The model under review builds one solid part; all positions refer to its coordinate system, in mm. A direction names the side the tool comes from. Coordinates: 2 decimals unless noted, no trailing zeros. Loops run counter-clockwise (first coordinate to the right, second up) from the corner with the lowest first, then second, coordinate; pieces in that order, holes last. Notation, with made-up numbers: M 39.25,-4.75 L 51.25,-4.75 A8 ccw 51.25,1.25 Z; hole C 14.25,-38.5 d3. An arc over 180 degrees is marked long. Use CSV: the item, a comma, the result in double quotes. Start each with the question number.
1. Tool access review of faces 4 (the cylindrical face through (-5.961, -26.846, 3.451)), 5 (the flat face through (12, -12, 0)), 6 (the cylindrical face through (10.382, -19.961, 4.535)): name each direction out of +Z, -Z, +X, -X, +Y, -Y from which nothing blocks a thin tool from reaching the whole face with its end or side.
2. Draft analysis for pull direction X (two halves, no side actions). For faces 1 (the flat face through (10, -10, 2)), 2 (the cylindrical face through (6.691, -12.864, -7.888)), 3 (the flat face through (-23, 0, 7)), state which applies: +X half, -X half, draft (parallel to the pull), parting line (faces both ways), or undercut.
3. Add section C-C, the plane z = -2.5. Write out the cut boundary in (x, y).
4. Clearance check with flat-ended pins moving along their axes: P1, Ø1.5, axis at x = 7.5, y = -12, coming from the +Z side; P2, Ø2, axis at y = 12.5, z = -6.5, coming from the -X side; P3, Ø2, axis at x = -20, y = 18, coming from the -Z side; P4, Ø16.5, axis at x = -8, y = -2.5, coming from the -Z side. State where each tip first meets the part, or that it passes through.
5. Add section D-D, the plane x = -18. Write out the cut boundary in (y, z), then the cut area to 3 significant figures.
6. For L1, parallel to Y at x = 0, z = 5.15; L2, parallel to Z at x = 21, y = 0.5; L3, parallel to Z at x = -14, y = 23.5, list the stretches that pass through material, from the lowest coordinate up.
7. Add section A-A, the plane y = 0. Write out the cut boundary in (x, z), then the cut area to 3 significant figures.
from build123d import *

# Parameters (mm, degrees)
SKETCH_R        = 27.5
PAD_DEPTH       = 7
SKETCH001_R     = 12.5
POCKET_DEPTH    = 7.001
SKETCH002_R     = 22.5
POCKET001_DEPTH = 5
SKETCH003_R     = 14.5
PAD001_DEPTH    = 16
SKETCH004_R     = 12.5
POCKET002_DEPTH = 23.001


with BuildPart() as part:
    # Sketch → Pad (new body)
    with BuildSketch(Plane.XY):
        Circle(SKETCH_R)
    extrude(amount=PAD_DEPTH)

    # Sketch001 (on Face3 of Pad) → Pocket (cut, through all)
    with BuildSketch(Plane.XY.offset(7)):
        Circle(SKETCH001_R)
    extrude(amount=-POCKET_DEPTH, mode=Mode.SUBTRACT)

    # Sketch002 (on Face3 of Pocket) → Pocket001 (cut)
    with BuildSketch(Plane.XY.offset(7)):
        Circle(SKETCH002_R)
    extrude(amount=-POCKET001_DEPTH, mode=Mode.SUBTRACT)

    # Sketch003 → Pad001 (join)
    with BuildSketch(Plane.XY):
        Circle(SKETCH003_R)
    extrude(amount=-PAD001_DEPTH)

    # Sketch004 (on Face6 of Pad001) → Pocket002 (cut, through all)
    with BuildSketch(Plane(origin=(0, 0, -16), x_dir=(1, 0, 0), z_dir=(0, 0, -1))):
        Circle(SKETCH004_R)
    extrude(amount=-POCKET002_DEPTH, mode=Mode.SUBTRACT)


solid = part.part
Computed:
1,face 4,"+Z, -Z"
1,face 5,"-Z"
1,face 6,"+Z"
2,face 1,"undercut"
2,face 2,"parting line"
2,face 3,"draft"
3,outline,"C 0,0 d29; hole C 0,0 d25"
4,P1,"stops at z = 2"
4,P2,"stops at x = -8.83"
4,P3,"stops at z = 0"
4,P4,"stops at z = -16"
5,outline,"M -20.79,0 L 20.79,0 L 20.79,7 L 13.5,7 L 13.5,2 L -13.5,2 L -13.5,7 L -20.79,7 Z"
5,area,"156 mm^2"
6,L1,"y = -27.5 to -22.5, 22.5 to 27.5"
6,L2,"z = 0 to 2"
6,L3,"z = 0 to 7"
7,outline,"M -27.5,0 L -14.5,0 L -14.5,-16 L -12.5,-16 L -12.5,2 L -22.5,2 L -22.5,7 L -27.5,7 Z; M 12.5,-16 L 14.5,-16 L 14.5,0 L 27.5,0 L 27.5,7 L 22.5,7 L 22.5,2 L 12.5,2 Z"
7,area,"174 mm^2"
